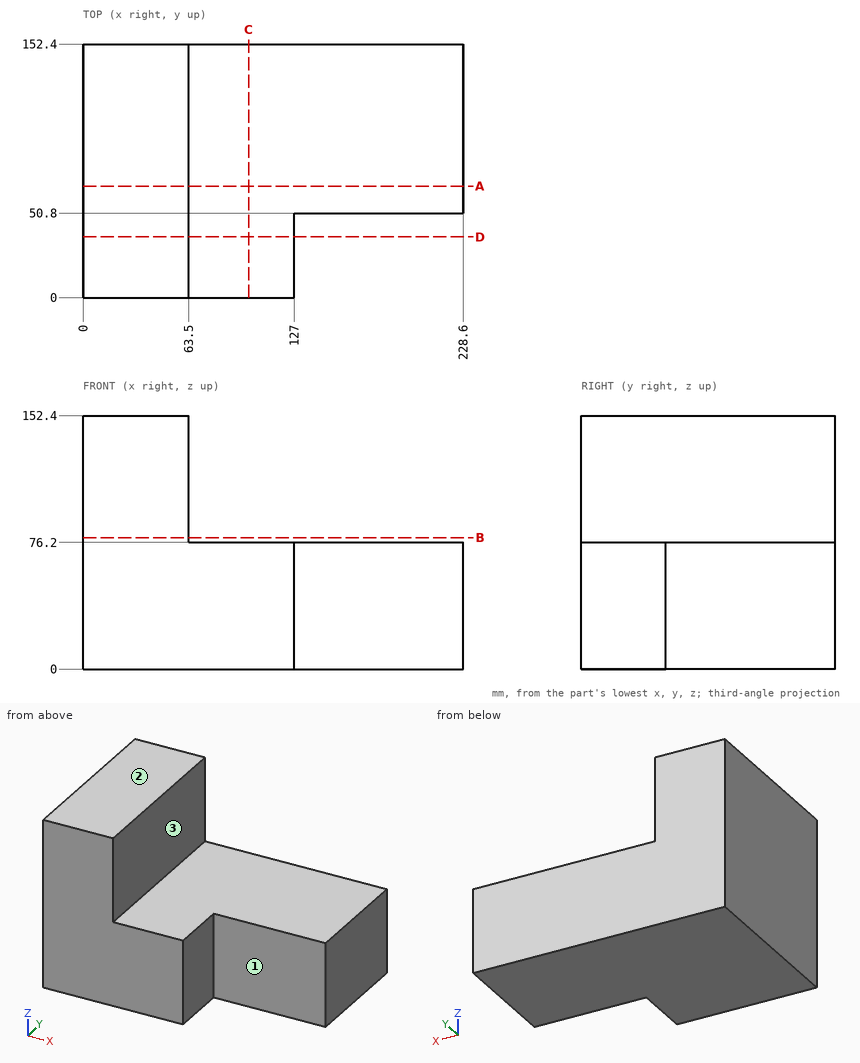
Design review of the part shown in the three views and the two pictorial views. Dimensions are in mm from the part's minimum x, y and z. A direction names the side the tool comes from. Coordinates: 2 decimals unless noted, no trailing zeros. Loops run counter-clockwise (first coordinate to the right, second up) from the corner with the lowest first, then second, coordinate; pieces in that order, holes last. Notation, with made-up numbers: (2.5, 57.5) - (19.5, 57.5) arc R14 cw to (19.5, 76.5) - close; hole circle Ø9 at (67.5, 8.5). An arc over 180 degrees is marked (long way). Use a Markdown table: item, result. Add a question column.
Item 1: We need section C-C (x = 99.5). Give the boundary of the cut face in (y, z), and give its area (3 significant figures).
Item 2: For line 1 (X direction, y = 120, z = 94.5); line 2 (Z direction, x = 124.5, y = 7); line 3 (Y direction, x = 211.5, z = 72.5), list the stretches that pass through material, from the lowest coordinate up.
Item 3: Insertion check: pin 1 Ø12 at (y, z) = (69, 87.5) entering from +X. The pin has a flat end and moves straight along its axis. Give the tip position at first contact, or say it passes through.
Item 4: We need section D-D (y = 36.5). Give the boundary of the cut face in (x, z), and give its area (3 significant figures).
Item 5: We need section A-A (y = 67). Give the boundary of the cut face in (x, z).
Item 6: Tool access review of the marked faces 1, 2 and 3: name each direction out of +Z, -Z, +X, -X, +Y, -Y from which nothing blocks a thin tool from reaching the whole face with its end or side.
Item 7: We need section B-B (z = 79). Give the boundary of the cut face in (x, y).
Results list:
| question | item | result |
|---|---|---|
| 1 | outline | (0, 0) - (152.4, 0) - (152.4, 76.2) - (0, 76.2) - close |
| 1 | area | 11,600 mm^2 |
| 2 | line 1 | x = 0 to 63.5 |
| 2 | line 2 | z = 0 to 76.2 |
| 2 | line 3 | y = 50.8 to 152.4 |
| 3 | pin 1 | stops at x = 63.5 |
| 4 | outline | (0, 0) - (127, 0) - (127, 76.2) - (63.5, 76.2) - (63.5, 152.4) - (0, 152.4) - close |
| 4 | area | 14,500 mm^2 |
| 5 | outline | (0, 0) - (228.6, 0) - (228.6, 76.2) - (63.5, 76.2) - (63.5, 152.4) - (0, 152.4) - close |
| 6 | face 1 | +Z, -Z, +X, -Y |
| 6 | face 2 | +Z, +X, -X, +Y, -Y |
| 6 | face 3 | +Z, +X, +Y, -Y |
| 7 | outline | (0, 0) - (63.5, 0) - (63.5, 152.4) - (0, 152.4) - close |
